Autodesk Inventor part; units mm, degrees
ref_plane "РабПлоскость1" through (0, 0, 60) normal (0, 0, 1) x (1, 0, 0)
ref_plane "РабПлоскость2" through (0, 70, 0) normal (0, 1, 0) x (-1, 0, 0)
ref_plane "YZ Plane" through (0, 0, 0) normal (1, 0, 0) x (0, 1, 0)
sketch "Эскиз1" plane through (0, 0, 0) normal (0, 0, 1) x (1, 0, 0)
  line L0 (-35.3564, 0.0006) -> (-0.0011, 35.3559)
  line L1 (-35.3564, 0.0006) -> (-0.0011, -35.3548)
  line L2 (-0.0011, -35.3548) -> (35.3543, 0.0006)
  line L3 (35.3543, 0.0006) -> (-0.0011, 35.3559)
  point P0 (0, 0)
  point P1 (0, 0)
sketch "Эскиз2" plane through (0, 0, 0) normal (0, 0, 1) x (1, 0, 0)
  point P0 (0, 0)
ref_plane "РабПлоскость1" through (0, 0, 60) normal (0, 0, 1) x (1, 0, 0)
sketch "Эскиз3" plane through (0, 0, 60) normal (0, 0, 1) x (1, 0, 0)
  line L0 (-17.6777, 0) -> (0, 17.6777)
  line L1 (0, 17.6777) -> (17.6777, 0)
  line L2 (17.6777, 0) -> (0, -17.6777)
  line L3 (0, -17.6777) -> (-17.6777, 0)
  point P0 (0, 0)
sketch "Эскиз4" plane through (0, 0, 60) normal (0, 0, 1) x (1, 0, 0)
  point P0 (0, 0)
sketch "Эскиз5" plane through (0, 0, 60) normal (0, 0, 1) x (1, 0, 0)
  point P0 (0, 0)
sketch "Эскиз6" plane through (0, 0, 0) normal (0, 0, 1) x (1, 0, 0)
  point P0 (0, 0)
sketch "Эскиз7" plane through (0, 0, 0) normal (0, 0, 1) x (1, 0, 0)
  point P0 (0, 0)
loft "Лофт1" add profiles "Эскиз1", "Эскиз3"
sketch "Эскиз8" plane through (0, 0, 0) normal (0, 1, 0) x (-1, 0, 0)
  point P0 (0, 0)
ref_plane "РабПлоскость2" through (0, 70, 0) normal (0, 1, 0) x (-1, 0, 0)
sketch "Эскиз9" plane through (0, 70, 0) normal (0, 1, 0) x (-1, 0, 0)
  line L0 (-9.9989, 45) -> (10.0011, 45)
  line L1 (10.0011, 45) -> (10.0011, 15)
  line L2 (10.0011, 15) -> (-9.9989, 15)
  line L3 (-9.9989, 15) -> (-9.9989, 45)
  line L4 (0.0011, 0) -> (-35.3543, 0)
  point P0 (0, 0)
extrude "Выдавливание1" cut sketch "Эскиз9" against normal blind 110
Model file for the job. Use its own axes, mm. A direction names the side the tool comes from. Give positions to 0.01 mm unless a question says otherwise; leave off trailing zeros. Answer as CSV lines item,"result".
1. 3-axis set-ups, long thin cutter, end or side, ignore diameter. For faces 1 (the face through (0, 0, 0)), 2 (the face through (0, 0, 15)): which of +Z, -Z, +X, -X, +Y, -Y reach the whole face in a straight line?
Responses:
face 1,"-Z, +X, -X, +Y, -Y"
face 2,"+Y, -Y"
2. Drill centre lines: L1, parallel to Z at x = -4.5, y = 8.5; L2, parallel to X at y = -10, z = 21; L3, parallel to X at y = -7, z = 34.5. Where is each one in solid material? Low to high. Write a range as [from, to].
Responses:
L1,"z = [0, 15], [45, 60]"
L2,"x = [-19.17, -10], [10, 19.17]"
L3,"x = [-18.19, -10], [10, 18.19]"
3. Pin check, flat tips, straight feed: pin 1 (3 mm diameter, centred on x = 16, z = 32.5, fed in from +Y); pin 2 (3 mm diameter, centred on x = 22.5, z = 40.5, fed in from -Y); pin 3 (4 mm diameter, centred on x = 25, z = 30.5, fed in from -Y). Stop position of each tip, or through.
Responses:
pin 1,"stops at y = 11.34"
pin 2,"stops at y = -2.49"
pin 3,"stops at y = -3.45"
4. Two-plate mould, pull along X, no slides. Class faces 3 (the face through (-10.001, 0, 30)), 4 (the face through (0, 0, 60)): +X half, -X half, draft (parallel to the pull), parting line (faces both ways), or undercut.
Responses:
face 3,"undercut"
face 4,"draft"
